Input: part model. Units: mm. Frame: model coordinates. Face numbers are marked on the shaded views. A direction names the side the tool comes from. Give positions to 0.01 mm unless a question says otherwise; leave off trailing zeros. Loops run counter-clockwise (first coordinate to the right, second up) from the corner with the lowest first, then second, coordinate; pieces in that order, holes last. Notation, with made-up numbers: M -18,85.5 L -14,85.5 A22 ccw -14,97.5 Z; hole C 7,67 d1. An arc over 180 degrees is marked long. Use a Markdown table: item, result. Add a question column.
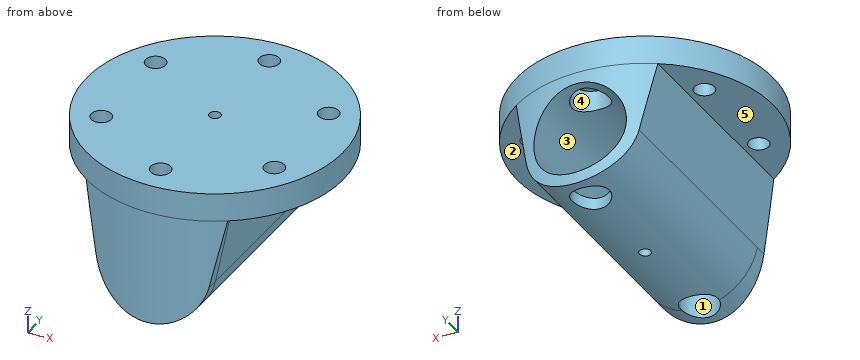
from build123d import *

# Parameters (mm, degrees)
SKETCH1_R                       = 22.4
BOSS_EXTRUDE1_DEPTH             = 5
BOSS_EXTRUDE2_REACH             = 34.071
BOSS_EXTRUDE2_END_RADIUS        = 22.4
SKETCH3_R                       = 8.1
BOSS_EXTRUDE2_DIRECTION_2_DEPTH = 18
BOSS_EXTRUDE5_START             = 21
BOSS_EXTRUDE5_DEPTH             = 21
CUT_EXTRUDE2_START              = -21
CUT_EXTRUDE2_DEPTH              = 21
SKETCH2_R                       = 1.75
CUT_EXTRUDE1_DEPTH              = 41.479130543
CUT_EXTRUDE3_DEPTH              = 21
CUT_EXTRUDE3_DEPTH_BACK         = 1.5
SKETCH7_R                       = 3.25
SKETCH7_R_2                     = 1.75
SKETCH8_R                       = 1
CUT_EXTRUDE4_DEPTH              = 41.479130543


with BuildPart() as part:
    # Sketch1 → Boss-Extrude1 (new body)
    with BuildSketch(Plane.XY):
        Circle(SKETCH1_R)
    extrude(amount=BOSS_EXTRUDE1_DEPTH)



with BuildPart() as body_2:
    # Boss-Extrude2: up to this cylinder (the profile starts inside it)
    boss_extrude2_end = Plane(origin=(0, 0, -6.007051), z_dir=(0, 0, -1)) * Cylinder(BOSS_EXTRUDE2_END_RADIUS, 113.942, mode=Mode.PRIVATE)
    # Sketch3 → Boss-Extrude2 (new, up to the surface)
    with BuildSketch(Plane(origin=(0, 0, 0), x_dir=(1, 0, 0), z_dir=(0, 1, 0)), mode=Mode.PRIVATE) as boss_extrude2_sk1:
        with BuildLine():
            Line((-9.89110529, 12.143535207), (-12.4, 0))
            Line((-12.4, 0), (12.4, 0))
            Line((12.4, 0), (9.89110529, 12.143535207))
            ThreePointArc((9.89110529, 12.143535207), (0, 20.2), (-9.89110529, 12.143535207))
        make_face()
        with Locations(Location((0, 10.1, 0), (0, 0, 270))):
            Circle(SKETCH3_R, mode=Mode.SUBTRACT)
    boss_extrude2_tool1 = extrude(boss_extrude2_sk1.sketch, amount=BOSS_EXTRUDE2_REACH, mode=Mode.PRIVATE) & boss_extrude2_end
    add(boss_extrude2_tool1.solids().sort_by_distance((-10.832312, 0, -6.007051))[0])

    # Sketch3 → Boss-Extrude2 direction 2 (add)
    with BuildSketch(Plane(origin=(0, 0, 0), x_dir=(1, 0, 0), z_dir=(0, 1, 0))):
        with BuildLine():
            Line((-9.89110529, 12.143535207), (-12.4, 0))
            Line((-12.4, 0), (12.4, 0))
            Line((12.4, 0), (9.89110529, 12.143535207))
            ThreePointArc((9.89110529, 12.143535207), (0, 20.2), (-9.89110529, 12.143535207))
        make_face()
        with Locations(Location((0, 10.1, 0), (0, 0, 270))):
            Circle(SKETCH3_R, mode=Mode.SUBTRACT)
    extrude(amount=-BOSS_EXTRUDE2_DIRECTION_2_DEPTH)


with BuildPart() as part_1:
    add(part.part)

    add(body_2.part)  # Boss-Extrude5 merges body 2
    # Sketch4 → Boss-Extrude5 (add)
    with BuildSketch(Plane(origin=(0, 0, 0), x_dir=(-1, 0, 0), z_dir=(0, 0, -1)).offset(BOSS_EXTRUDE5_START)):
        with BuildLine():
            Line((9.89110529, -18), (12.4, -18))
            Line((12.4, -18), (12.4, -18.654758106))
            ThreePointArc((12.4, -18.654758106), (0, -22.4), (-12.4, -18.654758106))
            Line((-12.4, -18.654758106), (-12.4, -18))
            Line((-12.4, -18), (-9.89110529, -18))
            Line((-9.89110529, -18), (9.89110529, -18))
        make_face()
    extrude(amount=-BOSS_EXTRUDE5_DEPTH)

    # Sketch6 → Cut-Extrude2 (cut)
    with BuildSketch(Plane(origin=(0, -18, 0), x_dir=(1, 0, 0), z_dir=(0, 1, 0)).offset(CUT_EXTRUDE2_START)):
        with BuildLine():
            Line((9.89110529, 12.143535207), (12.4, 0))
            Line((12.4, 0), (12.4, 21))
            Line((12.4, 21), (-12.4, 21))
            Line((-12.4, 21), (-12.4, 0))
            Line((-12.4, 0), (-9.89110529, 12.143535207))
            ThreePointArc((-9.89110529, 12.143535207), (0, 20.2), (9.89110529, 12.143535207))
        make_face()
    extrude(amount=CUT_EXTRUDE2_DEPTH, mode=Mode.SUBTRACT)

    # Sketch2 → Cut-Extrude1 (cut, through all)
    with BuildSketch(Plane.XY.offset(5)):
        with Locations((0, 17.5)):
            Circle(SKETCH2_R)
        with Locations((15.155444566, 8.75)):
            Circle(SKETCH2_R)
        with Locations((15.155444566, -8.75)):
            Circle(SKETCH2_R)
        with Locations((0, -17.5)):
            Circle(SKETCH2_R)
        with Locations((-15.155444566, -8.75)):
            Circle(SKETCH2_R)
        with Locations((-15.155444566, 8.75)):
            Circle(SKETCH2_R)
    extrude(amount=-CUT_EXTRUDE1_DEPTH, mode=Mode.SUBTRACT)

    # Sketch7 → Cut-Extrude3 (cut, two sides: drawn at the far end of the back side and taken through both)
    # profile 1 of 2: a face of its own
    with BuildSketch(Plane(origin=(0, 0, 0), x_dir=(-1, 0, 0), z_dir=(0, 0, -1)).offset(-CUT_EXTRUDE3_DEPTH_BACK)):
        with Locations(Location((0, 17.5, 0), (0, 0, 188.849872023))):
            Circle(SKETCH7_R)
        with Locations(Location((0, 17.5, 0), (0, 0, 180))):
            Circle(SKETCH7_R_2, mode=Mode.SUBTRACT)
    # profile 2 of 2: a face of its own
    with BuildSketch(Plane(origin=(0, 0, 0), x_dir=(-1, 0, 0), z_dir=(0, 0, -1)).offset(-CUT_EXTRUDE3_DEPTH_BACK)):
        with Locations(Location((0, -17.5, 0), (0, 0, 180))):
            Circle(SKETCH7_R)
        with Locations(Location((0, -17.5, 0), (0, 0, 180))):
            Circle(SKETCH7_R_2, mode=Mode.SUBTRACT)
    extrude(amount=CUT_EXTRUDE3_DEPTH + CUT_EXTRUDE3_DEPTH_BACK, mode=Mode.SUBTRACT)

    # Sketch8 → Cut-Extrude4 (cut, through all)
    with BuildSketch(Plane.XY.offset(5)):
        Circle(SKETCH8_R)
    extrude(amount=-CUT_EXTRUDE4_DEPTH, mode=Mode.SUBTRACT)


solid = part_1.part
1) Ray query, line 1 (Y direction, x = 0, z = 3.4); line 2 (Y direction, x = 0, z = -18.8); line 3 (Y direction, x = 1.5, z = 2). Return the intervals inside material, ascending. Write a range as [from, to].
2) Reachability of the marked faces 1, 2 and 3 from +Z, -Z, +X, -X, +Y, -Y: full face, straight path, thin tool, end or side. Return the list, or none.
3) Contact query for flat-ended pins moving along their axis: P1, Ø3, axis at x = -1.5, y = -19, coming from the -Z side; P2, Ø3, axis at x = -8, y = 17, coming from the -Z side; P3, Ø4, axis at x = -2.5, z = -7, coming from the +Y side; P4, Ø2, axis at x = 15.16, y = 8.75, coming from the +Z side. Output: stop coordinate, or through.
4) Section query D-D, the plane y = 8.75. Return the cut outline in (x, z), and give its area (3 significant figures).
5) Section query C-C, the plane z = -10.1. Return the cut outline in (x, y).
6) Section query B-B, the plane x = 14.5. Return the cut outline in (y, z), and give its area (3 significant figures).
7) Pull-direction query (Y, two-part tool) for the marked faces 4 and 5; classes: pulls with the +Y half, pulls with the -Y half, needs draft (parallel to the pull), parting line crosses it, or undercut.
8) Section query A-A, the plane y = -9.5. Return the cut outline in (x, z), and give its area (3 significant figures).
Entries:
| question | item | result |
|---|---|---|
| 1 | line 1 | y = [-22.4, -19.25], [-15.75, -1], [1, 15.75], [19.25, 22.4] |
| 1 | line 2 | y = [-22.4, -20.75], [-14.25, -1], [1, 14.25], [20.75, 22.4] |
| 1 | line 3 | y = [-22.35, -18.4], [-16.6, 16.6], [18.4, 22.35] |
| 2 | face 1 | -Z |
| 2 | face 2 | -Z, +X, +Y, -Y |
| 2 | face 3 | +Y |
| 3 | P1 | stops at z = -20.12 |
| 3 | P2 | stops at z = -17.83 |
| 3 | P3 | stops at y = -18 |
| 3 | P4 | passes through |
| 4 | outline | M -20.62,0 L -16.91,0 L -16.91,5 L -20.62,5 Z; M -13.41,0 L -12.4,0 L -9.89,-12.14 A10.1 ccw 9.89,-12.14 L 12.4,0 L 13.41,0 L 13.41,5 L -13.41,5 Z; M 16.91,0 L 20.62,0 L 20.62,5 L 16.91,5 Z; hole C 0,-10.1 d16.2 |
| 4 | area | 355 mm² |
| 5 | outline | M -10.31,-19.88 A22.4 ccw 10.31,-19.88 L 10.31,19.88 A22.4 ccw 8.1,20.88 L 8.1,-18 L 3.21,-18 A3.25 cw -3.21,-18 L -8.1,-18 L -8.1,20.88 A22.4 ccw -10.31,19.88 Z |
| 6 | outline | M -17.07,0 L -10.37,0 L -10.37,5 L -17.07,5 Z; M -7.13,0 L 7.13,0 L 7.13,5 L -7.13,5 Z; M 10.37,0 L 17.07,0 L 17.07,5 L 10.37,5 Z |
| 6 | area | 138 mm² |
| 7 | face 4 | undercut |
| 7 | face 5 | needs draft |
| 8 | outline | M -20.29,0 L -16.74,0 L -16.74,5 L -20.29,5 Z; M -13.57,0 L -12.4,0 L -9.89,-12.14 A10.1 ccw 9.89,-12.14 L 12.4,0 L 13.57,0 L 13.57,5 L -13.57,5 Z; M 16.74,0 L 20.29,0 L 20.29,5 L 16.74,5 Z; hole C 0,-10.1 d16.2 |
| 8 | area | 355 mm² |
